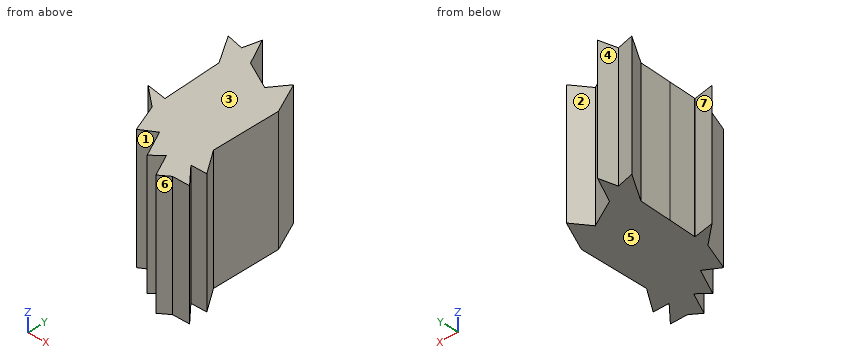
from build123d import *

# Parameters (mm, degrees)
F1_DEPTH = 254


with BuildPart() as f1:
    # F0 (on Top) → F1 (new body)
    with BuildSketch(Plane.XY):
        Polygon((-147.782792, -92.178449), (-146.70594, -121.784464), (-93.500725, -162.532108), (-44.075843, -200.384555), (-2.940414, -231.888456), (-1.797586, -141.762128), (0, 0), (-57.565849, 31.310931), (-116.964364, 63.618676), (-154.185936, 83.864048), (-152.300298, 32.021948), (-149.868549, -34.834455), (-147.822325, -91.091555), (-146.70594, -92.379923), align=None)
        Polygon((-190.108119, -84.259592), (-146.70594, -121.784464), (-147.782792, -92.178449), align=None)
        Polygon((-93.500725, -162.532108), (-146.70594, -121.784464), (-124.113187, -180.818781), align=None)
        Polygon((-44.075843, -200.384555), (-93.500725, -162.532108), (-65.873049, -219.272062), align=None)
        Polygon((-147.822325, -91.091555), (-147.782792, -92.178449), (-146.70594, -92.379923), align=None)
        Polygon((-2.940414, -231.888456), (-44.075843, -200.384555), (-20.746138, -248.582482), (0, -234.140396), align=None)
        Polygon((-1.797586, -141.762128), (-2.940414, -231.888456), (0, -234.140396), (35.582049, -234.591587), (0, -193.527976), (33.124767, -193.948008), align=None)
        Polygon((-190.108119, 92.880812), (-152.300298, 32.021948), (-154.185936, 83.864048), align=None)
        Polygon((-57.565849, 31.310931), (0, 0), (-30.732522, 66.347875), align=None)
        Polygon((-145.151658, 119.856003), (-154.185936, 83.864048), (-116.964364, 63.618676), align=None)
    extrude(amount=F1_DEPTH)


solid = f1.part
Model file for the job. Use its own axes, mm. Face numbers are marked on the shaded views. A direction names the side the tool comes from. Give positions to 0.01 mm unless a question says otherwise; leave off trailing zeros. Loops run counter-clockwise (first coordinate to the right, second up) from the corner with the lowest first, then second, coordinate; pieces in that order, holes last.
1) Tool access for the marked faces 1, 2 and 3: list every direction of +Z, -Z, +X, -X, +Y, -Y with a clear straight run to the whole face (end or side of a thin tool).
2) Saw through at B-B (z = 69). Write the cut outline in (x, y).
3) Saw through at C-C (x = -163.5). Write the cut outline in (y, z), plus the area to 3 significant figures.
4) Saw through at D-D (x = -81.5). Write the cut outline in (y, z), plus the area to 3 significant figures.
5) Flat gauge pins, fed straight in: pin 1 Ø1.5 at (x, z) = (-70, 192.5) entering from +Y; pin 2 Ø2 at (x, z) = (-82, 133) entering from -Y; pin 3 Ø1.5 at (x, z) = (-15, 37.5) entering from +Y. Where does each tip first touch, or does it go through?
6) Wall check: line 1 (Y direction, x = -177, z = 28.5); line 2 (Y direction, x = 16, z = 67.5); line 3 (X direction, y = -14, z = 186.5). Give the ranges that are in metal, low to high.
7) Saw through at A-A (y = -214). Write the cut outline in (x, z), plus the area to 3 significant figures.
8) Pull direction Y, two halves, no side cores. Call the marked faces 4, 5, 6 and 7: +Y half, -Y half, draft (parallel to the pull), parting line (faces both ways), or undercut.
Answer block:
1. face 1: +Z, -Z, -Y
1. face 2: +Z, -Z, +Y
1. face 3: +Z, +X, -X, +Y, -Y
2. outline: (-190.11, -84.26) - (-146.71, -121.78) - (-124.11, -180.82) - (-93.5, -162.53) - (-65.87, -219.27) - (-44.08, -200.38) - (-20.75, -248.58) - (0, -234.14) - (35.58, -234.59) - (0, -193.53) - (33.12, -193.95) - (-1.8, -141.76) - (0, 0) - (-30.73, 66.35) - (-57.57, 31.31) - (-116.96, 63.62) - (-145.15, 119.86) - (-154.19, 83.86) - (-190.11, 92.88) - (-152.3, 32.02) - (-147.82, -91.09) - (-147.78, -92.18) - close
3. outline: (-107.26, 0) - (-89.24, 0) - (-89.24, 254) - (-107.26, 254) - close; (50.05, 0) - (86.2, 0) - (86.2, 254) - (50.05, 254) - close
3. area: 13,800 mm2
4. outline: (-187.18, 0) - (44.33, 0) - (44.33, 254) - (-187.18, 254) - close
4. area: 58,800 mm2
5. pin 1: stops at y = 38.48
5. pin 2: stops at y = -188.21
5. pin 3: stops at y = 34
6. line 1: y = -95.59 to -86.71, 71.78 to 89.59
6. line 2: y = -234.34 to -211.99, -193.73 to -168.36
6. line 3: x = -150.63 to -0.18
7. outline: (-68.44, 0) - (-59.79, 0) - (-59.79, 254) - (-68.44, 254) - close; (-37.49, 0) - (17.74, 0) - (17.74, 254) - (-37.49, 254) - close
7. area: 16,200 mm2
8. face 4: +Y half
8. face 5: draft
8. face 6: -Y half
8. face 7: undercut
